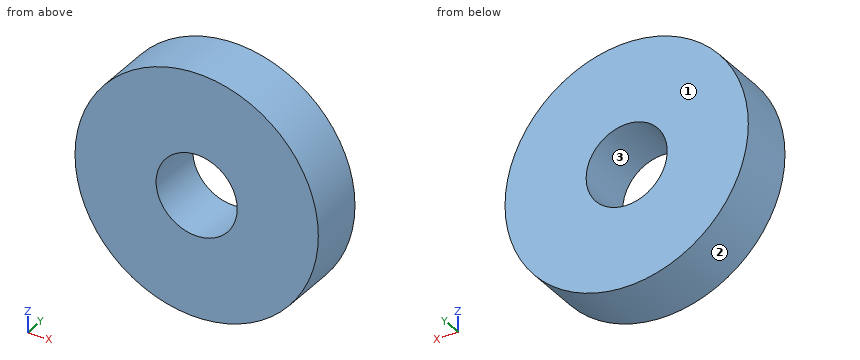
from build123d import *

# Parameters (mm, degrees)
CYLINDER013_R                = 3.5
CYLINDER013_DEPTH            = 10
CYLINDER012_R                = 10.5
CYLINDER012_DEPTH            = 5
CUT005014015_PLACEMENT_ANGLE = 90


with BuildPart() as cylinder013:
    # Cylinder013 → Cylinder013 (new body)
    with BuildSketch(Plane.XY.offset(-3)):
        Circle(CYLINDER013_R)
    extrude(amount=CYLINDER013_DEPTH)


with BuildPart() as obj1:
    # Cylinder012 → Cylinder012 (new body)
    with BuildSketch(Plane.XY):
        Circle(CYLINDER012_R)
    extrude(amount=CYLINDER012_DEPTH)

    # Cut005014015: cut Cylinder013
    add(cylinder013.part, mode=Mode.SUBTRACT)


with BuildPart() as obj1_1:
    # Cut005014015 placement: moved
    add(obj1.part.moved(Location((89, 0.5, 10.4))).rotate(Axis((89, 0.5, 10.4), (1, 0, 0)), CUT005014015_PLACEMENT_ANGLE))


solid = obj1_1.part
Design review of the part built by this model. Coordinates are the model's own, in mm. Face numbers are marked on the shaded views. Round coordinates to 2 decimals unless told otherwise and drop trailing zeros. Write each loop counter-clockwise with the first axis right and the second up, starting at its lowest first coordinate (ties: lowest second). Pieces come first, ordered by that corner, then holes. Notation, with made-up numbers: (63, 4.25) -> (119, 4.25) arc R34 ccw to (119, 39.25) -> close; hole circle Ø2 at (-6, 16). An arc over 180 degrees is marked (long way). One line per question, with ' | ' between items.
(1) Insertion check: P1, Ø2, axis at x = 95, y = -0.5, coming from the -Z side; P2, Ø5.5, axis at x = 89, z = 10.4, coming from the +Y side. Each pin has a flat end and moves straight along its axis. Give the tip position at first contact, or say it passes through.
Result sheet:
P1: z = 1.17 | P2: through
(2) Take a section at D-D, the plane x = 84. State the section outline as (y, z) points.
Result sheet:
outline: (-4.5, 1.17) -> (0.5, 1.17) -> (0.5, 19.63) -> (-4.5, 19.63) -> close
(3) Take a section at C-C, the plane y = -0.6. State the section outline as (x, z) points.
Result sheet:
outline: circle Ø21 at (89, 10.4); hole circle Ø7 at (89, 10.4)
(4) Draft analysis for pull direction X (two halves, no side actions). For the marked faces 1, 2 and 3, state which applies: released by +X, released by -X, zero draft, split by the parting line, or undercut.
Result sheet:
face 1: zero draft | face 2: split by the parting line | face 3: undercut
(5) Take a section at B-B, the plane z = 10.4. State the section outline as (x, y) points.
Result sheet:
outline: (78.5, -4.5) -> (85.5, -4.5) -> (85.5, 0.5) -> (78.5, 0.5) -> close; (92.5, -4.5) -> (99.5, -4.5) -> (99.5, 0.5) -> (92.5, 0.5) -> close
(6) Take a section at A-A, the plane x = 89. State the section outline as (y, z) points.
Result sheet:
outline: (-4.5, -0.1) -> (0.5, -0.1) -> (0.5, 6.9) -> (-4.5, 6.9) -> close; (-4.5, 13.9) -> (0.5, 13.9) -> (0.5, 20.9) -> (-4.5, 20.9) -> close
(7) Wall thickness on line 1 (Z direction, x = 89, y = -2.9); line 2 (X direction, y = -2.05, z = 12.5); line 3 (X direction, y = -0.45, z = 9.25): over which ranges is each line inside the solid? List them lowest first. Write a range as [from, to].
Result sheet:
line 1: [-0.1, 6.9], [13.9, 20.9] | line 2: [78.71, 86.2], [91.8, 99.29] | line 3: [78.56, 85.69], [92.31, 99.44]
